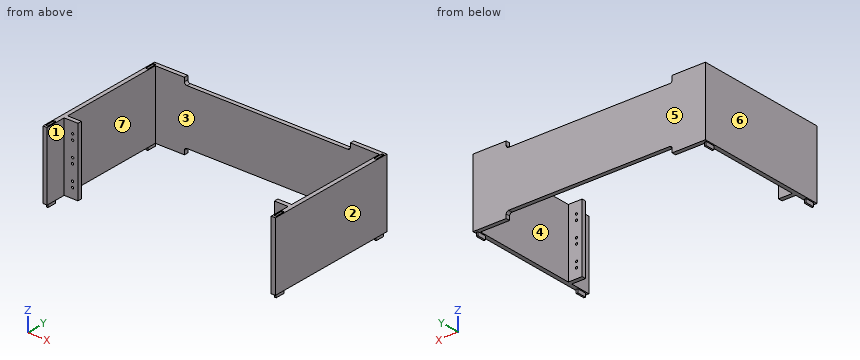
from build123d import *

# Parameters (mm, degrees)
F0_W          = 5
F0_H          = 1.5
F0_W_2        = 0.8
F0_H_2        = 3.5
F0_W_3        = 0.6
F0_H_3        = 3.3
F0_H_4        = 2.7
F0_H_5        = 0.6
F1_DEPTH      = 23
F1_DEPTH_BACK = 1.5
F3_D          = 0.8
F3_DEPTH      = 2
F3_TIP        = 0.2403442476
F5_D          = 0.8
F5_DEPTH      = 2
F5_TIP        = 0.2403442476
F6_DEPTH      = 2.8
F7_START      = 21.5
F7_DEPTH      = 1.5
F9_DEPTH      = 2


# Not quite as in the source:
# - a feature names something its author has since deleted; it is built from what else it names


with BuildPart() as f1:
    # F0 (on Top) → F1 (new body, two sides)
    with BuildSketch(Plane.XY) as f1_sk:
        with Locations((-38.0453250408, -14.9690947816)):
            Rectangle(F0_W, F0_H)
        Polygon((-42.0453250408, -23.1190947816), (-40.5453250408, -23.1190947816), (-40.5453250408, -15.7190947816), (-40.5453250408, -14.2190947816), (-40.5453250408, 23.8809052184), (-40.8953250408, 23.8809052184), (-40.8953250408, 21.0809052184), (-41.6953250408, 21.0809052184), (-41.6953250408, 23.8809052184), (-42.0453250408, 23.8809052184), align=None)
        with Locations((-41.2953250408, -20.5690947816)):
            Rectangle(F0_W_2, F0_H_2, mode=Mode.SUBTRACT)
        Polygon((-42.0453250408, 25.3809052184), (-42.0453250408, 23.8809052184), (-41.6953250408, 23.8809052184), (-41.6953250408, 24.5809052184), (-40.8953250408, 24.5809052184), (-40.8953250408, 23.8809052184), (-40.5453250408, 23.8809052184), (40.4546749592, 23.8809052184), (40.8046749592, 23.8809052184), (40.8046749592, 24.5809052184), (41.6046749592, 24.5809052184), (41.6046749592, 23.8809052184), (41.9546749592, 23.8809052184), (41.9546749592, 25.3809052184), align=None)
        Polygon((40.8046749592, 23.8809052184), (40.4546749592, 23.8809052184), (40.4546749592, -14.2186603174), (40.4546749592, -15.7186603174), (40.4546749592, -23.1190947816), (41.9546749592, -23.1190947816), (41.9546749592, 23.8809052184), (41.6046749592, 23.8809052184), (41.6046749592, 21.0809052184), (40.8046749592, 21.0809052184), align=None)
        with Locations((41.2046749592, -20.5690947816)):
            Rectangle(F0_W_2, F0_H_2, mode=Mode.SUBTRACT)
        with Locations((37.9546749592, -14.9686603174)):
            Rectangle(F0_W, F0_H)
        with Locations((-41.2953250408, -20.5690947816)):
            Rectangle(F0_W_2, F0_H_2)
        with Locations((-41.2953250408, -20.5690947816)):
            Rectangle(F0_W_3, F0_H_3, mode=Mode.SUBTRACT)
        with Locations((41.2046749592, -20.5690947816)):
            Rectangle(F0_W_2, F0_H_2)
        with Locations((41.2046749592, -20.5690947816)):
            Rectangle(F0_W_3, F0_H_3, mode=Mode.SUBTRACT)
        Polygon((40.9046749592, 23.8809052184), (40.8046749592, 23.8809052184), (40.8046749592, 21.0809052184), (41.6046749592, 21.0809052184), (41.6046749592, 23.8809052184), (41.5046749592, 23.8809052184), (41.5046749592, 21.1809052184), (40.9046749592, 21.1809052184), align=None)
        Polygon((40.8046749592, 24.5809052184), (40.8046749592, 23.8809052184), (40.9046749592, 23.8809052184), (40.9046749592, 24.4809052184), (41.5046749592, 24.4809052184), (41.5046749592, 23.8809052184), (41.6046749592, 23.8809052184), (41.6046749592, 24.5809052184), align=None)
        Polygon((-41.6953250408, 24.5809052184), (-41.6953250408, 23.8809052184), (-41.5953250408, 23.8809052184), (-41.5953250408, 24.4809052184), (-40.9953250408, 24.4809052184), (-40.9953250408, 23.8809052184), (-40.8953250408, 23.8809052184), (-40.8953250408, 24.5809052184), align=None)
        Polygon((-41.5953250408, 23.8809052184), (-41.6953250408, 23.8809052184), (-41.6953250408, 21.0809052184), (-40.8953250408, 21.0809052184), (-40.8953250408, 23.8809052184), (-40.9953250408, 23.8809052184), (-40.9953250408, 21.1809052184), (-41.5953250408, 21.1809052184), align=None)
        with Locations((-41.2953250408, -20.5690947816)):
            Rectangle(F0_W_3, F0_H_3)
        with Locations((-41.2953250408, 22.5309052184)):
            Rectangle(F0_W_3, F0_H_4)
        with Locations((41.2046749592, -20.5690947816)):
            Rectangle(F0_W_3, F0_H_3)
        with Locations((41.2046749592, 22.5309052184)):
            Rectangle(F0_W_3, F0_H_4)
        with Locations((41.2046749592, 24.1809052184)):
            Rectangle(F0_W_3, F0_H_5)
        with Locations((-41.2953250408, 24.1809052184)):
            Rectangle(F0_W_3, F0_H_5)
    extrude(amount=F1_DEPTH)
    extrude(f1_sk.sketch, amount=-F1_DEPTH_BACK)

    # F3
    with Locations(Plane.XZ.offset(15.7190947816)):
        with Locations((-37.4758429825, 18.9999998622), (-37.4758429825, 16.9999998622), (-37.4758429825, 11.4999998622), (-37.5126936273, 9.5), (-37.5126936273, 3.9999998622), (-37.5126936273, 2)):
            Hole(F3_D / 2, depth=F3_DEPTH)
            with Locations((0, 0, -(F3_DEPTH + F3_TIP / 2))):  # 118° drill point
                Cone(0, F3_D / 2, F3_TIP, mode=Mode.SUBTRACT)

    # F5
    with Locations(Plane.XZ.offset(15.7186603174)):
        with Locations((37.5221328411, 19.00000019), (37.5221328411, 17.00000019), (37.5221328411, 11.50000019), (37.4725908041, 9.5000003278), (37.4725908041, 4.00000019), (37.4725908041, 2.0000003278)):
            Hole(F5_D / 2, depth=F5_DEPTH)
            with Locations((0, 0, -(F5_DEPTH + F5_TIP / 2))):  # 118° drill point
                Cone(0, F5_D / 2, F5_TIP, mode=Mode.SUBTRACT)

    # F0 (on Top) → F6 (join)
    with BuildSketch(Plane.XY):
        with Locations((-41.2953250408, 22.5309052184)):
            Rectangle(F0_W_3, F0_H_4)
        with Locations((-41.2953250408, 24.1809052184)):
            Rectangle(F0_W_3, F0_H_5)
        with Locations((-41.2953250408, -20.5690947816)):
            Rectangle(F0_W_3, F0_H_3)
        with Locations((41.2046749592, 22.5309052184)):
            Rectangle(F0_W_3, F0_H_4)
        with Locations((41.2046749592, 24.1809052184)):
            Rectangle(F0_W_3, F0_H_5)
        with Locations((41.2046749592, -20.5690947816)):
            Rectangle(F0_W_3, F0_H_3)
    extrude(amount=-F6_DEPTH)

    # F0 (on Top) → F7 (cut)
    with BuildSketch(Plane.XY.offset(F7_START)):
        with Locations((-41.2953250408, -20.5690947816)):
            Rectangle(F0_W_2, F0_H_2)
        with Locations((-41.2953250408, -20.5690947816)):
            Rectangle(F0_W_3, F0_H_3, mode=Mode.SUBTRACT)
        with Locations((41.2046749592, -20.5690947816)):
            Rectangle(F0_W_2, F0_H_2)
        with Locations((41.2046749592, -20.5690947816)):
            Rectangle(F0_W_3, F0_H_3, mode=Mode.SUBTRACT)
        with Locations((-41.2953250408, -20.5690947816)):
            Rectangle(F0_W_3, F0_H_3)
        with Locations((41.2046749592, -20.5690947816)):
            Rectangle(F0_W_3, F0_H_3)
        with Locations((-41.2953250408, 22.5309052184)):
            Rectangle(F0_W_3, F0_H_4)
        with Locations((41.2046749592, 22.5309052184)):
            Rectangle(F0_W_3, F0_H_4)
        Polygon((-41.5953250408, 23.8809052184), (-41.6953250408, 23.8809052184), (-41.6953250408, 21.0809052184), (-40.8953250408, 21.0809052184), (-40.8953250408, 23.8809052184), (-40.9953250408, 23.8809052184), (-40.9953250408, 21.1809052184), (-41.5953250408, 21.1809052184), align=None)
        Polygon((40.9046749592, 23.8809052184), (40.8046749592, 23.8809052184), (40.8046749592, 21.0809052184), (41.6046749592, 21.0809052184), (41.6046749592, 23.8809052184), (41.5046749592, 23.8809052184), (41.5046749592, 21.1809052184), (40.9046749592, 21.1809052184), align=None)
        with Locations((-41.2953250408, 24.1809052184)):
            Rectangle(F0_W_3, F0_H_5)
        with Locations((41.2046749592, 24.1809052184)):
            Rectangle(F0_W_3, F0_H_5)
        Polygon((40.8046749592, 24.5809052184), (40.8046749592, 23.8809052184), (40.9046749592, 23.8809052184), (40.9046749592, 24.4809052184), (41.5046749592, 24.4809052184), (41.5046749592, 23.8809052184), (41.6046749592, 23.8809052184), (41.6046749592, 24.5809052184), align=None)
        Polygon((-41.6953250408, 24.5809052184), (-41.6953250408, 23.8809052184), (-41.5953250408, 23.8809052184), (-41.5953250408, 24.4809052184), (-40.9953250408, 24.4809052184), (-40.9953250408, 23.8809052184), (-40.8953250408, 23.8809052184), (-40.8953250408, 24.5809052184), align=None)
    extrude(amount=F7_DEPTH, mode=Mode.SUBTRACT)

    # F8 (on face) → F9 (cut)
    with BuildSketch(Plane(origin=(0, 25.3809052184, 0), x_dir=(-1, 0, 0), z_dir=(0, 1, 0))):
        with BuildLine():
            ThreePointArc((-29.9546749592, 21.5864117908), (-29.6910710623, 20.9500156878), (-29.0546749592, 20.6864117908))
            Line((-29.0546749592, 20.6864117908), (29.1453250408, 20.6864117908))
            ThreePointArc((29.1453250408, 20.6864117908), (29.7817211439, 20.9500156878), (30.0453250408, 21.5864117908))
            Line((30.0453250408, 21.5864117908), (30.0453250408, 23))
            Line((30.0453250408, 23), (-29.9546749592, 23))
            Line((-29.9546749592, 23), (-29.9546749592, 21.5864117908))
        make_face()
        with BuildLine():
            Line((-29.9546749592, -0.0864118039), (-29.9546749592, -1.500000013))
            Line((-29.9546749592, -1.500000013), (30.0453250408, -1.500000013))
            Line((30.0453250408, -1.500000013), (30.0453250408, -0.0864118039))
            ThreePointArc((30.0453250408, -0.0864118039), (29.7817211439, 0.5499842992), (29.1453250408, 0.8135881961))
            Line((29.1453250408, 0.8135881961), (-29.0546749592, 0.8135881961))
            ThreePointArc((-29.0546749592, 0.8135881961), (-29.6910710623, 0.5499842992), (-29.9546749592, -0.0864118039))
        make_face()
    extrude(amount=-F9_DEPTH, mode=Mode.SUBTRACT)


solid = f1.part
Build history of the part. All positions in model axes, mm. Face numbers are marked on the shaded views. A direction names the side the tool comes from. Round coordinates to 2 decimals unless told otherwise and drop trailing zeros. Write each loop counter-clockwise with the first axis right and the second up, starting at its lowest first coordinate (ties: lowest second). Pieces come first, ordered by that corner, then holes. Notation, with made-up numbers: M 48.25,29.25 L 106.25,29.25 A33 ccw 106.25,68.25 Z; hole C 71.25,-26.5 d1. An arc over 180 degrees is marked long. Answer in a Markdown table with one row per item.
1. Which spindle directions (+Z, -Z, +X, -X, +Y, -Y) get a long thin tool onto all of the face, cutting with end or side? Do the marked faces 1, 2 and 3. Say none if no direction does.
Geometry check:
| item | result |
|---|---|
| face 1 | +Z, -Z, -Y |
| face 2 | +Z, -Z, +X, +Y, -Y |
| face 3 | +Z, -Z |
2. Flat gauge pins, fed straight in: P1, Ø1.4, axis at y = 22.5, z = -2.5, coming from the -X side; P2, Ø6, axis at x = -0.5, z = 14, coming from the -Y side; P3, Ø0.6, axis at y = -21.5, z = -2, coming from the +X side. Where does each tip first touch, or does it go through?
Geometry check:
| item | result |
|---|---|
| P1 | x = -41.6 |
| P2 | y = 23.88 |
| P3 | x = 41.5 |
3. Saw through at B-B (z = 6.75). List the corners of the cut face in (x, y).
Geometry check:
| item | result |
|---|---|
| outline | M -42.05,-23.12 L -40.55,-23.12 L -40.55,-15.72 L -35.55,-15.72 L -35.55,-14.22 L -40.55,-14.22 L -40.55,23.88 L 40.45,23.88 L 40.45,-14.22 L 35.45,-14.22 L 35.45,-15.72 L 40.45,-15.72 L 40.45,-23.12 L 41.95,-23.12 L 41.95,25.38 L -42.05,25.38 Z |
4. Saw through at A-A (y = 4.5). List the corners of the cut face in (x, z), and give its area (3 significant figures).
Geometry check:
| item | result |
|---|---|
| outline | M -42.05,-1.5 L -40.55,-1.5 L -40.55,23 L -42.05,23 Z; M 40.45,-1.5 L 41.95,-1.5 L 41.95,23 L 40.45,23 Z |
| area | 73.5 mm2 |
5. Mould opens along Y. For the marked faces 4, 5, 6 and 7 say: +Y half, -Y half, draft (parallel to the pull), parting line (faces both ways), or undercut.
Geometry check:
| item | result |
|---|---|
| face 4 | undercut |
| face 5 | +Y half |
| face 6 | draft |
| face 7 | undercut |
6. Probe L1, parallel to X at y = -0.5, z = 21; L2, parallel to Y at x = 36.5, z = 9; L3, parallel to Y at x = -14, z = 12.5. List the from-to ranges inside material, lowest first. Write a range as [from, to].
Geometry check:
| item | result |
|---|---|
| L1 | [-42.05, -40.55], [40.45, 41.95] |
| L2 | [-15.72, -14.22], [23.88, 25.38] |
| L3 | [23.88, 25.38] |
7. Saw through at C-C (x = -0.5). List the corners of the cut face in (y, z).
Geometry check:
| item | result |
|---|---|
| outline | M 23.88,0.81 L 25.38,0.81 L 25.38,20.69 L 23.88,20.69 Z |
